The listing builds one solid part. Answer for the finished solid, in the listing's coordinates (mm). A direction names the side the tool comes from. Round coordinates to 2 decimals unless told otherwise and drop trailing zeros. Write each loop counter-clockwise with the first axis right and the second up, starting at its lowest first coordinate (ties: lowest second). Pieces come first, ordered by that corner, then holes. Notation, with made-up numbers: M 24,13.25 L 75,13.25 A13 ccw 75,20.25 Z; hole C -15,53 d7. An arc over 180 degrees is marked long. Answer as CSV lines item,"result". Start each with the question number.
from build123d import *

# Parameters (mm, degrees)
BOSS_EXTRUDE1_DEPTH                                 = 12.7
SKETCH2_W                                           = 15.9004
SKETCH2_H                                           = 12.7
CUT_EXTRUDE1_DEPTH                                  = 1
CUT_EXTRUDE1_DEPTH_BACK                             = 153.4
CBORE_FOR_00_BINDING_HEAD_MACHINE_SCREW_D           = 12.7
CBORE_FOR_00_BINDING_HEAD_MACHINE_SCREW_CBORE_D     = 29.718
CBORE_FOR_00_BINDING_HEAD_MACHINE_SCREW_CBORE_DEPTH = 19.7104
LPATTERN1_COUNT                                     = 2
LPATTERN1_PITCH                                     = 44.45
LPATTERN1_COUNT_DIR2                                = 2
LPATTERN1_PITCH_DIR2                                = 19.05


with BuildPart() as part:
    # Sketch1 → Boss-Extrude1 (new body, symmetric)
    with BuildSketch(Plane.XY):
        with BuildLine():
            Line((0, 0), (0, 127))
            ThreePointArc((0, 127), (-7.439487758, 144.960512242), (-25.4, 152.4))
            Line((-25.4, 152.4), (-88.9, 152.4))
            Line((-88.9, 152.4), (-88.9, 101.6))
            Line((-88.9, 101.6), (-35.052, 101.6))
            ThreePointArc((-35.052, 101.6), (-28.227005348, 98.772994652), (-25.4, 91.948))
            Line((-25.4, 91.948), (-25.4, 0))
            Line((-25.4, 0), (0, 0))
        make_face()
    extrude(amount=BOSS_EXTRUDE1_DEPTH, both=True)

    # Sketch2 → Cut-Extrude1 (cut, two sides)
    with BuildSketch(Plane(origin=(0, 152.4, 0), x_dir=(1, 0, 0), z_dir=(0, 1, 0))) as cut_extrude1_sk:
        with Locations((-80.9498, 0)):
            Rectangle(SKETCH2_W, SKETCH2_H)
    extrude(amount=CUT_EXTRUDE1_DEPTH, mode=Mode.SUBTRACT)
    extrude(cut_extrude1_sk.sketch, amount=-CUT_EXTRUDE1_DEPTH_BACK, mode=Mode.SUBTRACT)

    # CBORE for #00 Binding Head Machine Screw1 (through all)
    with Locations(Plane.XY.offset(12.7)):
        with Locations((-61.976, 127)):
            CounterBoreHole(CBORE_FOR_00_BINDING_HEAD_MACHINE_SCREW_D / 2, CBORE_FOR_00_BINDING_HEAD_MACHINE_SCREW_CBORE_D / 2, CBORE_FOR_00_BINDING_HEAD_MACHINE_SCREW_CBORE_DEPTH)

    # Sketch7 → CBORE for 3/8 Socket Head Cap Screw1 (revolve, cut)
    with BuildSketch(Plane(origin=(0, 12.7, 0), x_dir=(0, 0, -1), z_dir=(0, 1, 0))):
        Polygon((0, 0), (0, 88.9), (5.0419, 88.9), (5.0419, 9.700511387), (5.334, 9.525), (7.9375, 9.525), (7.9375, 0), align=None)
    revolve(axis=Axis((6.35, 12.7, 0), (-1, 0, 0)), mode=Mode.SUBTRACT)

    # Sketch9 → #8-32 Tapped Hole1 (revolve, cut)
    with BuildSketch(Plane(origin=(-88.9, 104.775, -9.525), x_dir=(0, 0, 1), z_dir=(0, 1, 0))):
        Polygon((0, 0), (0, 9.927806461), (1.7272, 8.89), (1.7272, 0), align=None)
    f_8_32_tapped_hole1 = revolve(axis=Axis((-95.25, 104.775, -9.525), (1, 0, 0)), mode=Mode.SUBTRACT)

    # LPattern1: 8-32 Tapped Hole1 2 × 2
    with Locations(*[(0, i * LPATTERN1_PITCH, j * LPATTERN1_PITCH_DIR2) for i in range(LPATTERN1_COUNT) for j in range(LPATTERN1_COUNT_DIR2) if (i, j) != (0, 0)]):
        add(f_8_32_tapped_hole1, mode=Mode.SUBTRACT)


solid = part.part
Q1. Find section C-C (x = -38). Determine the outline of the cut face in (y, z).
Q2. For faces 5 (the face through (-59, 121, -7.01)), 6 (the face through (-81, 127, 6.35)), 7 (the face through (-84.517, 103.062, 9.3)), 8 (the face through (-4.7, 4.83, 1.03)), determine the directions among +Z, -Z, +X, -X, +Y, -Y from which every point of the face is accessible in a straight line to the end or side of a thin tool.
Q3. Straight lines are drawn through the part: L1, parallel to Y at x = -41.5, z = 9.25; L2, parallel to Y at x = -71.5, z = -6.25; L3, parallel to X at y = 16.5, z = -4.5 (3 decimals). For each, find the intervals that lie inside material, in ascending order.
Q4. Each of these flat-tipped pins is pushed along its axis until it touches: P1, Ø14.5, axis at x = -61.976, y = 127, coming from the +Z side; P2, Ø2, axis at y = 104.775, z = 9.525, coming from the +X side; P3, Ø1.5, axis at x = -42, z = -10, coming from the -Y side; P4, Ø5, axis at y = 9, z = 1, coming from the +X side (3 decimals). Where does it stop, or does it pass through?
Q5. The mould has two halves that part along Y. Classify faces 1 (the face through (-57, 152.4, 0)), 2 (the face through (-28.302, 98.848, 0.178)), 3 (the face through (-73, 145, 0)), 4 (the face through (-79.152, 148.972, -9.364)): +Y half, -Y half, draft (parallel to the pull), parting line (faces both ways), or undercut.
Q6. Find section D-D (y = 84). Determine the outline of the cut face in (x, z).
Reported:
1,outline,"M 101.6,-12.7 L 152.4,-12.7 L 152.4,12.7 L 101.6,12.7 Z"
2,face 5,"+Z"
2,face 6,"-X, +Y, -Y"
2,face 7,"-X"
2,face 8,"+X"
3,L1,"y = 101.6 to 152.4"
3,L2,"y = 101.6 to 115.59, 138.41 to 152.4"
3,L3,"x = -25.4 to -9.525"
4,P1,"stops at z = -7.01"
4,P2,"stops at x = 0"
4,P3,"stops at y = 101.6"
4,P4,"stops at x = -9.525"
5,face 1,"+Y half"
5,face 2,"-Y half"
5,face 3,"draft"
5,face 4,"undercut"
6,outline,"M -25.4,-12.7 L 0,-12.7 L 0,12.7 L -25.4,12.7 Z"
